For this review, take the finished solid that the model builds, in its own axes (mm). Round coordinates to 2 decimals unless told otherwise and drop trailing zeros. Write each loop counter-clockwise with the first axis right and the second up, starting at its lowest first coordinate (ties: lowest second). Pieces come first, ordered by that corner, then holes. Notation, with made-up numbers: M 27.5,18.5 L 44.5,18.5 A13 cw 44.5,29.5 Z; hole C -34.5,78 d8. An arc over 180 degrees is marked long. One line per question, with ' | ' between items.
```python
from build123d import *

# Parameters (mm, degrees)
AUFSATZ_LINEAR_AUSTRAGEN1_DEPTH = 1000


with BuildPart() as part:
    # Skizze1 → Aufsatz-Linear austragen1 (new body)
    with BuildSketch(Plane(origin=(0, 0, 0), x_dir=(0, 0, -1), z_dir=(1, 0, 0))):
        with BuildLine():
            Line((0, 0), (1000, 0))
            Line((1000, 0), (1000, 2000))
            ThreePointArc((1000, 2000), (884.950154707, 1963.595638995), (811.783470431, 1867.635330981))
            Line((811.783470431, 1867.635330981), (188.216529569, 132.364669019))
            ThreePointArc((188.216529569, 132.364669019), (115.049845293, 36.404361005), (0, 0))
        make_face()
    extrude(amount=AUFSATZ_LINEAR_AUSTRAGEN1_DEPTH)


solid = part.part
```
Item 1: Take a section at B-B (y = 360). Write out the cut boundary in (x, z), then the cut area to 3 significant figures.
Results:
outline: M 0,-1000 L 1000,-1000 L 1000,-270.02 L 0,-270.02 Z | area: 730,000 mm2
Item 2: Take a section at C-C (z = -718.5). Write out the cut boundary in (x, y), then the cut area to 3 significant figures.
Results:
outline: M 0,0 L 1000,0 L 1000,1608.04 L 0,1608.04 Z | area: 1,610,000 mm2
Item 3: To check wall thickness, follow line 1 along Y through (x, z) = (54.5, -51); line 2 along Z through (x, y) = (827.5, 1411.5); line 3 along Y through (x, z) = (196.5, -122). State the ranges of each line that lie inside material, in increasing order. Write a range as from..to.
Results:
line 1: 0..6.61 | line 2: -1000..-647.87 | line 3: 0..41.52
Item 4: Take a section at A-A (x = 127). Write out the cut boundary in (y, z), then the cut area to 3 significant figures.
Results:
outline: M 0,-1000 L 2000,-1000 A200 ccw 1867.64,-811.78 L 132.36,-188.22 A200 cw 0,0 Z | area: 1,000,000 mm2
Item 5: Insertion check: pin 1 Ø1.5 at (x, z) = (809, -161) entering from +Y. The pin has a flat end and moves straight along its axis. Give the tip position at first contact, or say it passes through.
Results:
pin 1: y = 82.37
